Geometry check sheet. Reference: the model listing, model coordinates, mm. A direction names the side the tool comes from. Round coordinates to 2 decimals unless told otherwise and drop trailing zeros. Order: outer loops, then holes, each group sorted by start corner. A loop starts at its lowest first (then second) coordinate and runs counter-clockwise, first axis right, second up. Notation, with made-up numbers: (-2.5, 75) - (31.5, 75) arc R24 ccw to (31.5, 87) - close; hole circle Ø10 at (-7.75, 86). An arc over 180 degrees is marked (long way). Write each question's results on one line, items separated by ' | '.
Autodesk Inventor part; units mm, degrees
ref_plane "YZ Plane" through (0, 0, 0) normal (1, 0, 0) x (0, 1, 0)
ref_plane "XZ Plane" through (0, 0, 0) normal (0, 1, 0) x (-1, 0, 0)
ref_plane "XY Plane" through (0, 0, 0) normal (0, 0, 1) x (1, 0, 0)
sketch "Sketch1" plane through (0, 0, 0) normal (0, 0, 1) x (1, 0, 0)
  line L0 (0, 26.1238) -> (688.34, 26.1238)
  line L1 (688.34, 26.1238) -> (688.34, -814.6162)
  line L2 (0, 26.1238) -> (0, -814.6162)
  line L3 (0, -814.6162) -> (167.64, -814.6162)
  line L4 (688.34, -814.6162) -> (520.7, -814.6162)
  line L5 (520.7, -890.8162) -> (764.54, -890.8162)
  line L6 (764.54, -890.8162) -> (764.54, 102.3238)
  line L7 (764.54, 102.3238) -> (-76.2, 102.3238)
  line L8 (-76.2, 102.3238) -> (-76.2, -890.8162)
  line L9 (-76.2, -890.8162) -> (167.64, -890.8162)
  line L10 (167.64, -814.6162) -> (167.64, -890.8162)
  line L11 (520.7, -814.6162) -> (520.7, -890.8162)
  point P0 (0, 0)
  dimension "d0" = 688.34
  dimension "d1" = 840.74
  dimension "d2" = 167.64
  dimension "d3" = 167.64
  dimension "d4" = 76.2
extrude "Extrusion1" add sketch "Sketch1" along normal blind 88.9
fillet "Fillet1" radius 19.05 18 edges at (-76.2, -394.2462, 88.9) (45.72, -890.8162, 88.9) (45.72, -890.8162, 0) (-76.2, -394.2462, 0) (-76.2, -890.8162, 44.45) (167.64, -890.8162, 44.45) (520.7, -890.8162, 44.45) (764.54, -890.8162, 44.45) (642.62, -890.8162, 88.9) (642.62, -890.8162, 0) (764.54, -394.2462, 88.9) (764.54, -394.2462, 0) (764.54, 102.3238, 44.45) (344.17, 102.3238, 88.9) (344.17, 102.3238, 0) (-76.2, 102.3238, 44.45) (520.7, -814.6162, 44.45) (167.64, -814.6162, 44.45)
sketch "Sketch2" plane through (764.54, -871.7662, 19.05) normal (1, 0, 0) x (0, 0, -1)
  line L0 (-65.2441, 154.6268) -> (-65.2441, 182.3935) construction
  line L1 (-65.2441, 182.3935) -> (47.3065, 182.3935) construction
  line L2 (47.3065, 182.3935) -> (47.3065, 154.6268) construction
  line L3 (47.3065, 154.6268) -> (-65.2441, 154.6268) construction
  line L4 (-58.9935, 771.5963) -> (-58.9935, 799.363) construction
  line L5 (-58.9935, 799.363) -> (53.557, 799.363) construction
  line L6 (53.557, 799.363) -> (53.557, 771.5963) construction
  line L7 (53.557, 771.5963) -> (-58.9935, 771.5963) construction
  point P0 (19.05, 871.7662)
  dimension "d3" = 167.64
sketch "Sketch3" plane through (-76.2, -871.7662, 19.05) normal (-1, 0, 0) x (0, 0, 1)
  line L0 (66.8415, 917.1452) -> (66.8415, 824.847) construction
  line L1 (66.8415, 824.847) -> (-3.0085, 824.847) construction
  line L2 (-3.0085, 824.847) -> (-3.0085, 917.1452) construction
  line L3 (-3.0085, 917.1452) -> (66.8415, 917.1452) construction
  line L4 (68.429, 179.765) -> (68.429, 87.4668) construction
  line L5 (68.429, 87.4668) -> (-1.421, 87.4668) construction
  line L6 (-1.421, 87.4668) -> (-1.421, 179.765) construction
  line L7 (-1.421, 179.765) -> (68.429, 179.765) construction
  point P0 (-19.05, 871.7662)
  dimension "d3" = 167.64
properties part number "Bumpers" material "Fabric"
(1) Access from +Z, -Z, +X, -X, +Y, -Y to the whole of each face (thin tool, end or side, straight path). Record for faces 1 (the face through (520.7, -852, 44)), 2 (the face through (-14, -357, 0)), 3 (the face through (615, -814.616, 44)).
Answers follow:
face 1: +Z, -Z, -Y | face 2: -Z, +X, -X, +Y, -Y | face 3: +Z, -Z
(2) Draft check along Y on faces 4 (the face through (-14, -357, 88.9)), 5 (the face through (44, -890.816, 44)), 6 (the face through (688.34, -388, 44)), 7 (the face through (350, 102.324, 44)). Enter one of: released by +Y, released by -Y, zero draft, split by the parting line, or undercut.
Answers follow:
face 4: zero draft | face 5: released by -Y | face 6: undercut | face 7: released by +Y
(3) Section check D-D (x = 236). Record the cut outline in (y, z).
Answers follow:
outline: (26.12, 0) - (83.27, 0) arc R19.05 ccw to (102.32, 19.05) - (102.32, 69.85) arc R19.05 ccw to (83.27, 88.9) - (26.12, 88.9) - close
(4) Depth check by flat-ended pin: pin 1 Ø1 at (x, z) = (280, 68) entering from -Y; pin 2 Ø1 at (y, z) = (-79, 74) entering from +X; pin 3 Ø8 at (y, z) = (-319.5, 12) entering from +X. Enter the tip coordinate at first touch or a pass-through.
Answers follow:
pin 1: y = 26.12 | pin 2: x = 764.19 | pin 3: x = 764.29
(5) Section check A-A (y = -563). Record the cut outline in (x, z), then the cut area to 3 significant figures.
Answers follow:
outline: (-76.2, 19.05) arc R19.05 ccw to (-57.15, 0) - (0, 0) - (0, 88.9) - (-57.15, 88.9) arc R19.05 ccw to (-76.2, 69.85) - close; (688.34, 0) - (745.49, 0) arc R19.05 ccw to (764.54, 19.05) - (764.54, 69.85) arc R19.05 ccw to (745.49, 88.9) - (688.34, 88.9) - close | area: 13,200 mm²
(6) Section check B-B (x = 49). Record the cut outline in (y, z), then the cut area to 3 significant figures.
Answers follow:
outline: (-890.82, 19.05) arc R19.05 ccw to (-871.77, 0) - (-814.62, 0) - (-814.62, 88.9) - (-871.77, 88.9) arc R19.05 ccw to (-890.82, 69.85) - close; (26.12, 0) - (83.27, 0) arc R19.05 ccw to (102.32, 19.05) - (102.32, 69.85) arc R19.05 ccw to (83.27, 88.9) - (26.12, 88.9) - close | area: 13,200 mm²
(7) Section check C-C (z = 47.5). Record the cut outline in (x, y).
Answers follow:
outline: (-76.2, -871.77) arc R19.05 ccw to (-57.15, -890.82) - (148.59, -890.82) arc R19.05 ccw to (167.64, -871.77) - (167.64, -833.67) arc R19.05 ccw to (148.59, -814.62) - (0, -814.62) - (0, 26.12) - (688.34, 26.12) - (688.34, -814.62) - (539.75, -814.62) arc R19.05 ccw to (520.7, -833.67) - (520.7, -871.77) arc R19.05 ccw to (539.75, -890.82) - (745.49, -890.82) arc R19.05 ccw to (764.54, -871.77) - (764.54, 83.27) arc R19.05 ccw to (745.49, 102.32) - (-57.15, 102.32) arc R19.05 ccw to (-76.2, 83.27) - close
(8) Material ranges on line 1 (X direction, y = -766, z = 29); line 2 (Y direction, x = 7, z = 25.5); line 3 (Y direction, x = 537.5, z = 65.5), recorded low to high.
Answers follow:
line 1: -76.2 to 0, 688.34 to 764.54 | line 2: -890.82 to -814.62, 26.12 to 102.32 | line 3: -890.68 to -814.75, 26.12 to 102.32
